```python
from build123d import *

# Parameters (mm, degrees)
SKETCH1_R               = 1
BOSS_EXTRUDE1_DEPTH     = 2
SKETCH4_W               = 2
SKETCH4_H               = 2
BOSS_EXTRUDE2_DEPTH     = 11
CUT_EXTRUDE1_DEPTH      = 13.903487901
CUT_EXTRUDE1_DEPTH_BACK = 13.903487901
CUT_EXTRUDE2_DEPTH      = 14.133925537
CUT_EXTRUDE2_DEPTH_BACK = 14.133925537
CUT_EXTRUDE3_DEPTH      = 14.133925537
CUT_EXTRUDE3_DEPTH_BACK = 14.133925537
SKETCH7_R               = 0.5


with BuildPart() as part:
    # Sketch1 → Boss-Extrude1 (new body)
    with BuildSketch(Plane(origin=(0, 0, 0), x_dir=(1, 0, 0), z_dir=(0, 1, 0))):
        with BuildLine():
            Line((-10, 2.5), (0, 2.5))
            Line((0, 2.5), (0, -2.5))
            Line((0, -2.5), (-10, -2.5))
            ThreePointArc((-10, -2.5), (-12.5, 0), (-10, 2.5))
        make_face()
        with Locations(Location((-10, 0, 0), (0, 0, 270))):
            Circle(SKETCH1_R, mode=Mode.SUBTRACT)
    extrude(amount=BOSS_EXTRUDE1_DEPTH)

    # Sketch4 → Boss-Extrude2 (add)
    with BuildSketch(Plane(origin=(0, 0, 0), x_dir=(0, 0, -1), z_dir=(1, 0, 0))):
        with Locations((0, 1)):
            Rectangle(SKETCH4_W, SKETCH4_H)
    extrude(amount=BOSS_EXTRUDE2_DEPTH)

    # Sketch5 → Cut-Extrude1 (cut, two sides: drawn at the far end of the back side and taken through both)
    with BuildSketch(Plane(origin=(0, 2, 0), x_dir=(1, 0, 0), z_dir=(0, 1, 0)).offset(-CUT_EXTRUDE1_DEPTH_BACK)):
        with BuildLine():
            Line((10, 1), (10, 1.5))
            Line((10, 1.5), (12, 1.5))
            Line((12, 1.5), (12, -1.5))
            Line((12, -1.5), (10, -1.5))
            Line((10, -1.5), (10, -1))
            ThreePointArc((10, -1), (11, 0), (10, 1))
        make_face()
    extrude(amount=CUT_EXTRUDE1_DEPTH + CUT_EXTRUDE1_DEPTH_BACK, mode=Mode.SUBTRACT)

    # Sketch6 → Cut-Extrude2 (cut, two sides: drawn at the far end of the back side and taken through both)
    with BuildSketch(Plane(origin=(0, 0, -1), x_dir=(-1, 0, 0), z_dir=(0, 0, -1)).offset(-CUT_EXTRUDE2_DEPTH_BACK)):
        with BuildLine():
            Line((-10, 2), (-10, 2.5))
            Line((-10, 2.5), (-12, 2.5))
            Line((-12, 2.5), (-12, -0.5))
            Line((-12, -0.5), (-10, -0.5))
            Line((-10, -0.5), (-10, 0))
            ThreePointArc((-10, 0), (-11, 1), (-10, 2))
        make_face()
    extrude(amount=CUT_EXTRUDE2_DEPTH + CUT_EXTRUDE2_DEPTH_BACK, mode=Mode.SUBTRACT)

    # Sketch7 → Cut-Extrude3 (cut, two sides: drawn at the far end of the back side and taken through both)
    with BuildSketch(Plane(origin=(0, 0, -1), x_dir=(-1, 0, 0), z_dir=(0, 0, -1)).offset(-CUT_EXTRUDE3_DEPTH_BACK)):
        with Locations(Location((-10, 1, 0), (0, 0, 90))):
            Circle(SKETCH7_R)
    extrude(amount=CUT_EXTRUDE3_DEPTH + CUT_EXTRUDE3_DEPTH_BACK, mode=Mode.SUBTRACT)


solid = part.part
```
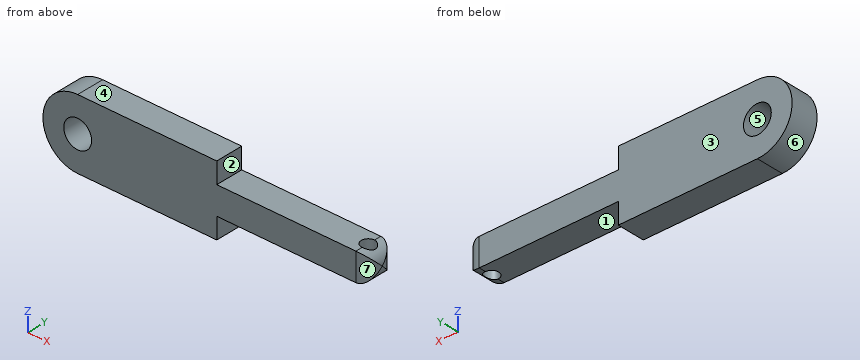
Part model, mm, in its own coordinate system. Face numbers are marked on the shaded views. A direction names the side the tool comes from. Give positions to 0.01 mm unless a question says otherwise; leave off trailing zeros. Write each loop counter-clockwise with the first axis right and the second up, starting at its lowest first coordinate (ties: lowest second). Pieces come first, ordered by that corner, then holes. Notation, with made-up numbers: (-31, 17.5) -> (-4, 17.5) arc R25 ccw to (-4, 35.5) -> close; hole circle Ø3 at (2.25, 48). An arc over 180 degrees is marked (long way). Put each result on its own line as item: value. Start each with the question number.
Item 1: Cut at C-C (x = -9.5). List the corners of the cut face in (y, z), then the cut area to 3 significant figures.
Item 2: Cut at D-D (x = 7). List the corners of the cut face in (y, z), then the cut area to 3 significant figures.
Item 3: Cut at A-A (y = 1.8). List the corners of the cut face in (x, z).
Item 4: Pull direction X, two halves, no side cores. Call the marked faces 4, 5, 6 and 7: pulls with the +X half, pulls with the -X half, needs draft (parallel to the pull), parting line crosses it, or undercut.
Item 5: Pin check, flat tip, straight feed: pin 1 Ø0.8 at (y, z) = (1, -2) entering from +X. Stop position of the tip, or through.
Item 6: Which spindle directions (+Z, -Z, +X, -X, +Y, -Y) get a long thin tool onto all of the face, cutting with end or side? Do the marked faces 1, 2 and 3. Say none if no direction does.
Item 7: Wall check: L1, parallel to X at y = 0.95, z = 0; L2, parallel to Y at x = 10, z = 0; L3, parallel to X at y = 1.3, z = 0.4. Give the ranges that are in metal, low to high. Write a range as [from, to].
Item 8: Cut at B-B (z = -0.35). List the corners of the cut face in (x, y).
Answer list:
1. outline: (0, -2.5) -> (2, -2.5) -> (2, -0.87) -> (0, -0.87) -> close; (0, 0.87) -> (2, 0.87) -> (2, 2.5) -> (0, 2.5) -> close
1. area: 6.54 mm2
2. outline: (0, -1) -> (2, -1) -> (2, 1) -> (0, 1) -> close
2. area: 4.00 mm2
3. outline: (-10, -2.5) -> (0, -2.5) -> (0, -1) -> (10, -1) arc R1 ccw to (10.6, -0.8) -> (10.6, 0.8) arc R1 ccw to (10, 1) -> (0, 1) -> (0, 2.5) -> (-10, 2.5) arc R2.5 ccw to start; hole circle Ø2 at (-10, 0)
4. face 4: needs draft
4. face 5: undercut
4. face 6: pulls with the -X half
4. face 7: pulls with the +X half
5. pin 1: stops at x = 0
6. face 1: -Z, +X, +Y, -Y
6. face 2: +Z, +X, +Y, -Y
6. face 3: +Z, -Z, +X, -X, +Y
7. L1: x = [-12.5, -11], [-9, 9.5], [10.5, 11]
7. L2: y = [0, 0.5], [1.5, 2]
7. L3: x = [-12.47, -10.92], [-9.08, 9.6], [10.4, 10.92]
8. outline: (-12.48, 0) -> (-10.94, 0) -> (-10.94, 2) -> (-12.48, 2) -> close; (-9.06, 0) -> (10, 0) arc R1 ccw to (10.94, 0.65) -> (10.94, 1.35) arc R1 ccw to (10, 2) -> (-9.06, 2) -> close; hole circle Ø1 at (10, 1)
